The model under review builds one solid part; all positions refer to its coordinate system, in mm. A direction names the side the tool comes from. Coordinates: 2 decimals unless noted, no trailing zeros. Write each loop counter-clockwise with the first axis right and the second up, starting at its lowest first coordinate (ties: lowest second). Pieces come first, ordered by that corner, then holes. Notation, with made-up numbers: (10.25, 30) - (60.25, 30) arc R32 ccw to (60.25, 59) - close; hole circle Ø10 at (80.25, 27). An arc over 180 degrees is marked (long way). Use one line per item in the form item = value. Start each with the question number.
```python
from build123d import *

# Parameters (mm, degrees)
BOSS_EXTRUDE1_DEPTH               = 9.5504
SKETCH2_R                         = 13.6144
BOSS_EXTRUDE2_DEPTH               = 1.1938
SKETCH3_R                         = 1.4732
CUT_EXTRUDE1_DEPTH                = 68.553783128
F_4_40_TAPPED_HOLE1_D             = 2.2606
F_1_4_28_TAPPED_HOLE1_D           = 5.4102
F_1_4_28_TAPPED_HOLE1_CSINK_D     = 7.366
F_1_4_28_TAPPED_HOLE1_CSINK_ANGLE = 82
SKETCH11_R                        = 3.175
CUT_EXTRUDE3_DEPTH                = 68.553783128
SKETCH12_R                        = 3.175
CUT_EXTRUDE4_DEPTH                = 3.175
LPATTERN1_COUNT                   = 2
LPATTERN1_PITCH                   = 15.875


with BuildPart() as part:
    # Sketch1 → Boss-Extrude1 (new body)
    with BuildSketch(Plane(origin=(0, 0, 0), x_dir=(1, 0, 0), z_dir=(0, 1, 0))):
        with BuildLine():
            Line((0, 0), (31.75, 0))
            ThreePointArc((31.75, 0), (52.3875, 20.6375), (31.75, 41.275))
            Line((31.75, 41.275), (0, 41.275))
            Line((0, 41.275), (0, 0))
        make_face()
    extrude(amount=BOSS_EXTRUDE1_DEPTH)

    # Sketch2 → Boss-Extrude2 (add)
    with BuildSketch(Plane(origin=(0, 9.5504, 0), x_dir=(1, 0, 0), z_dir=(0, 1, 0))):
        with Locations(Location((31.75, 20.6375, 0), (0, 0, 270))):
            Circle(SKETCH2_R)
    extrude(amount=BOSS_EXTRUDE2_DEPTH)

    # Sketch3 → Cut-Extrude1 (cut, through all)
    with BuildSketch(Plane(origin=(0, 10.7442, 0), x_dir=(1, 0, 0), z_dir=(0, 1, 0))):
        with Locations(Location((23.2156, 35.4203, 0), (0, 0, 270))):
            Circle(SKETCH3_R)
        with Locations(Location((48.8188, 20.6375, 0), (0, 0, 270))):
            Circle(SKETCH3_R)
        with Locations(Location((23.2156, 5.8547, 0), (0, 0, 270))):
            Circle(SKETCH3_R)
    extrude(amount=-CUT_EXTRUDE1_DEPTH, mode=Mode.SUBTRACT)

    # #4-40 Tapped Hole1 (through all)
    with Locations(Plane(origin=(0, 0, 0), x_dir=(-1, 0, 0), z_dir=(0, -1, 0))):
        with Locations((-12.7, 5.9436), (-12.7, 35.3314)):
            Hole(F_4_40_TAPPED_HOLE1_D / 2)

    # 1/4-28 Tapped Hole1 (through all)
    with Locations(Plane(origin=(0, 0, 0), x_dir=(-1, 0, 0), z_dir=(0, -1, 0))):
        with Locations((-31.75, 20.6375)):
            CounterSinkHole(F_1_4_28_TAPPED_HOLE1_D / 2, F_1_4_28_TAPPED_HOLE1_CSINK_D / 2, counter_sink_angle=F_1_4_28_TAPPED_HOLE1_CSINK_ANGLE)

    # Sketch11 → Cut-Extrude3 (cut, through all)
    with BuildSketch(Plane(origin=(0, 0, 0), x_dir=(0, 0, 1), z_dir=(0.499999999999998, 0.8660254037844398, 0))):
        with Locations(Location((-20.6375, 14.25807156, 0), (0, 0, 270))):
            Circle(SKETCH11_R)
    extrude(amount=CUT_EXTRUDE3_DEPTH, mode=Mode.SUBTRACT)

    # Sketch12 → Cut-Extrude4 (cut)
    with BuildSketch(Plane.XZ):
        with Locations(Location((31.75, -20.6375, 0), (0, 0, 270))):
            Circle(SKETCH12_R)
    extrude(amount=-CUT_EXTRUDE4_DEPTH, mode=Mode.SUBTRACT)

    # Sketch15 → #6-32 Tapped Hole1 (revolve, cut)
    with BuildSketch(Plane(origin=(0, 4.7752, -28.575), x_dir=(0, 0, 1), z_dir=(0, 1, 0))):
        Polygon((0, 0), (0, 10.33769403), (1.35255, 9.525), (1.35255, 0), align=None)
    f_6_32_tapped_hole1 = revolve(axis=Axis((-6.35, 4.7752, -28.575), (1, 0, 0)), mode=Mode.SUBTRACT)

    # LPattern1: #6-32 Tapped Hole1 ×2
    with Locations(*[(0, 0, i * LPATTERN1_PITCH) for i in range(1, LPATTERN1_COUNT)]):
        add(f_6_32_tapped_hole1, mode=Mode.SUBTRACT)


solid = part.part
```
1. For faces 1 (the flat face through (35, 10.744, -21)), 2 (the cylindrical face through (45.25, 10.14, -22.41)), list the 3-axis set-ups (+Z, -Z, +X, -X, +Y, -Y) from which the entire face can be reached by the end or side of a thin tool; tool diameter is ignored.
2. For P1, Ø10, axis at x = 31.75, z = -20.64, coming from the -Y side; P2, Ø2.5, axis at x = 48.82, z = -20.64, coming from the -Y side; P3, Ø1, axis at x = 41, y = 3, coming from the -Z side; P4, Ø2.5, axis at y = 4.78, z = -28.58, coming from the +X side, all flat-tipped, find the tip position at first contact; note any pin that passes through.
3. Take a section at A-A (x = 5). State the section outline as (y, z) points (3 decimals).
4. The part is to be moulded in two halves that separate along X. For faces 3 (the cylindrical face through (4.696, 3.434, -28.751)), 4 (the cylindrical face through (52.383, 4.708, -20.184)), 5 (the cylindrical face through (22.319, 4.842, -7.024)), 6 (the cylindrical face through (28.65, 1.86, -19.95)), say which applies: released by +X, released by -X, zero draft, split by the parting line, or undercut.
5. Take a section at C-C (y = 8.75). Count the separate pieces of the cut face and the enclosed holes in it, plus the area to 3 significant figures.
6. For L1, parallel to X at y = 1.25, z = -36; L2, parallel to Y at x = 3.25, z = -12.7; L3, parallel to Z at x = 21.5, y = 9.25 (3 decimals), list the stretches that pass through material, from the lowest coordinate up.
7. Take a section at B-B (z = -16). State the section outline as (x, y) points, plus the area to 3 significant figures.
Returned:
q1.face_1 = +Z, -Z, +X, -X, +Y
q1.face_2 = +Y
q2.P1 = 0
q2.P2 = through
q2.P3 = -39.33
q2.P4 = 51.27
q3.outline = (0, -41.275) - (9.55, -41.275) - (9.55, 0) - (0, 0) - close; hole circle Ø2.705 at (4.775, -28.575); hole circle Ø2.705 at (4.775, -12.7)
q4.face_3 = zero draft
q4.face_4 = released by +X
q4.face_5 = undercut
q4.face_6 = undercut
q5.separate_pieces = 1
q5.enclosed_holes = 7
q5.area = 1,890 mm²
q6.L1 = 0 to 11.79, 13.61 to 21.86, 24.57 to 45.53
q6.L2 = 0 to 3.42, 6.13 to 9.55
q6.L3 = -41.275 to -23.802, -17.473 to 0
q7.outline = (0, 0) - (51.86, 0) - (51.86, 9.55) - (44.55, 9.55) - (44.55, 10.74) - (18.95, 10.74) - (18.95, 9.55) - (0, 9.55) - close
q7.area = 526 mm²
